```python
from build123d import *

# Parameters (mm, degrees)
SKETCH_2_W                = 25
SKETCH_2_H                = 25
EXTRUDE_2_DEPTH           = 20
SKETCH_8_W                = 17
SKETCH_8_H                = 7
CUT_EXTRUDE_5_DEPTH       = 10
CUT_EXTRUDE_6_DEPTH       = 12
SKETCH_13_W               = 20
SKETCH_13_H               = 0.2
CUT_EXTRUDE_7_DEPTH       = 12.5
HOLE_WIZARD_1_D           = 5.5
HOLE_WIZARD_1_DEPTH       = 16
HOLE_WIZARD_1_CBORE_D     = 9.5
HOLE_WIZARD_1_CBORE_DEPTH = 5.5
M5X0_8_1_D                = 4.2
M5X0_8_1_DEPTH            = 12.4
M5X0_8_1_TIP              = 1.2618073
SKETCH_16_R               = 4
CUT_EXTRUDE_8_DEPTH       = 35.369317712
SKETCH_17_R               = 2.75
CUT_EXTRUDE_9_DEPTH       = 6


with BuildPart() as part:
    # 草图2 → 凸台-拉伸2 (new, symmetric)
    with BuildSketch(Plane(origin=(0, 0, 0), x_dir=(0, 0, -1), z_dir=(1, 0, 0))):
        with Locations((0, 12.5)):
            Rectangle(SKETCH_2_W, SKETCH_2_H)
    extrude(amount=EXTRUDE_2_DEPTH, both=True)

    # 草图8 → 切除-拉伸5 (cut)
    with BuildSketch(Plane(origin=(20, 0, 0), x_dir=(0, 0, -1), z_dir=(1, 0, 0))):
        with Locations((-4, 9.5)):
            Rectangle(SKETCH_8_W, SKETCH_8_H)
    cut_extrude_5 = extrude(amount=-CUT_EXTRUDE_5_DEPTH, mode=Mode.SUBTRACT)

    # 镜向1: 切除-拉伸5 across plane
    add(cut_extrude_5.mirror(Plane(origin=(0, 0, 0), x_dir=(0, 0, 1), z_dir=(1, 0, 0))), mode=Mode.SUBTRACT)

    # 草图12 → 切除-拉伸6 (cut)
    with BuildSketch(Plane(origin=(0, 25, 0), x_dir=(1, 0, 0), z_dir=(0, 1, 0))):
        Polygon((-20, 4.5), (-7, 4.5), (-7, 0), (7, 0), (7, 4.5), (20, 4.5), (20, 3.5), (8, 3.5), (8, -1), (-8, -1), (-8, 3.5), (-20, 3.5), align=None)
    extrude(amount=-CUT_EXTRUDE_6_DEPTH, mode=Mode.SUBTRACT)

    # 草图13 → 切除-拉伸7 (cut)
    with BuildSketch(Plane.XY.offset(12.5)):
        with Locations((0, 12.9)):
            Rectangle(SKETCH_13_W, SKETCH_13_H)
    extrude(amount=-CUT_EXTRUDE_7_DEPTH, mode=Mode.SUBTRACT)

    # 孔1
    with Locations(Plane.XY.offset(12.5)):
        with Locations((-13.5, 19), (13.5, 19)):
            CounterBoreHole(HOLE_WIZARD_1_D / 2, HOLE_WIZARD_1_CBORE_D / 2, HOLE_WIZARD_1_CBORE_DEPTH, depth=HOLE_WIZARD_1_DEPTH)

    # M5x0.8 螺纹孔1
    with Locations(Plane.XY.offset(-4.5)):
        with Locations((-13.5, 19), (13.5, 19)):
            Hole(M5X0_8_1_D / 2, depth=M5X0_8_1_DEPTH)
            with Locations((0, 0, -(M5X0_8_1_DEPTH + M5X0_8_1_TIP / 2))):  # 118° drill point
                Cone(0, M5X0_8_1_D / 2, M5X0_8_1_TIP, mode=Mode.SUBTRACT)

    # 草图16 → 切除-拉伸8 (cut, through all)
    with BuildSketch(Plane(origin=(0, 25, 0), x_dir=(1, 0, 0), z_dir=(0, 1, 0))):
        with Locations(Location((0, 0, 0), (0, 0, 270))):
            Circle(SKETCH_16_R)
    extrude(amount=-CUT_EXTRUDE_8_DEPTH, mode=Mode.SUBTRACT)

    # 草图17 → 切除-拉伸9 (cut)
    with BuildSketch(Plane.XZ):
        with Locations(Location((-15, 0, 0), (0, 0, 270))):
            Circle(SKETCH_17_R)
        with Locations(Location((15, 0, 0), (0, 0, 270))):
            Circle(SKETCH_17_R)
    extrude(amount=-CUT_EXTRUDE_9_DEPTH, mode=Mode.SUBTRACT)


solid = part.part
```
Design review of the part built by this model. Coordinates are the model's own, in mm. A direction names the side the tool comes from. Round coordinates to 2 decimals unless told otherwise and drop trailing zeros. Order: outer loops, then holes, each group sorted by start corner. A loop starts at its lowest first (then second) coordinate and runs counter-clockwise, first axis right, second up. Notation, with made-up numbers: M 60.25,-30 L 119.25,-30 A30 cw 119.25,-7 Z; hole C 15.5,3 d6. An arc over 180 degrees is marked long. Put each result on its own line as item: value.
Q1. To check wall thickness, follow line 1 (Y direction, x = -13.5, z = 2.75); line 2 (Y direction, x = 13.5, z = 8.8); line 3 (Z direction, x = 5, y = 20.75). State the ranges of each line that lie inside material, in increasing order.
Reported:
line 1: 0 to 6, 13 to 16.25, 21.75 to 25
line 2: 0 to 6, 13 to 14.25, 23.75 to 25
line 3: -12.5 to 0, 1 to 12.5
Q2. Machinability: for faces 1 (the face through (-14, 15, -4.5)), 2 (the face through (6, 19, 1)), 3 (the face through (17, 19, -3.5)), 4 (the face through (-11, 17, 7)), 5 (the face through (0, 12.8, 6)), which of the approach directions +Z, -Z, +X, -X, +Y, -Y give a long, thin tool a straight path to every point of the face, cutting with its end or side? Answer none if there is none.
Reported:
face 1: -X, +Y
face 2: +Y
face 3: +X, +Y
face 4: +Z
face 5: +Z, +X, -X
Q3. Draft analysis for pull direction X (two halves, no side actions). For faces 6 (the face through (0, 19, 4)), 7 (the face through (-6, 19, 0)), 8 (the face through (5, 0, 0)), 9 (the face through (-20, 10, -5)), state which applies: released by +X, released by -X, zero draft, split by the parting line, or undercut.
Reported:
face 6: undercut
face 7: undercut
face 8: zero draft
face 9: released by -X
Q4. Consider section A-A (x = 0). State the section outline as (y, z) points.
Reported:
outline: M 0,-12.5 L 25,-12.5 L 25,-4 L 0,-4 Z; M 0,4 L 12.8,4 L 12.8,12.5 L 0,12.5 Z; M 13,4 L 25,4 L 25,12.5 L 13,12.5 Z
Q5. Consider section D-D (x = 5). State the section outline as (y, z) points, and give its area (4 significant figures).
Reported:
outline: M 0,-12.5 L 25,-12.5 L 25,0 L 12.8,0 L 12.8,12.5 L 0,12.5 Z; M 13,1 L 25,1 L 25,12.5 L 13,12.5 Z
area: 610.5 mm²
Q6. Consider section C-C (y = 7.5). State the section outline as (x, z) points, and give its area (3 significant figures).
Reported:
outline: M -20,-12.5 L 20,-12.5 L 20,-4.5 L 10,-4.5 L 10,12.5 L -10,12.5 L -10,-4.5 L -20,-4.5 Z; hole C 0,0 d8
area: 610 mm²
Q7. Consider section B-B (z = 8). State the section outline as (x, y) points, and give its area (3 significant figures).
Reported:
outline: M -20,0 L 20,0 L 20,6 L 10,6 L 10,12.8 L -10,12.8 L -10,6 L -20,6 Z; M -20,13 L 20,13 L 20,25 L -20,25 Z; hole C -13.5,19 d9.5; hole C 13.5,19 d9.5
area: 714 mm²
Q8. Insertion check: pin 1 Ø14.5 at (x, y) = (-15, 20) entering from +Z; pin 2 Ø2 at (y, z) = (10.5, 4) entering from -X; pin 3 Ø3 at (x, y) = (15.5, 17.5) entering from +Z. Each pin has a flat end and moves straight along its axis. Give the tip position at first contact, or say it passes through.
Reported:
pin 1: z = 12.5
pin 2: x = -10
pin 3: z = 7
